```python
from build123d import *

# Parameters (mm, degrees)
SKETCH1_W           = 20
SKETCH1_H           = 20
BOSS_EXTRUDE1_DEPTH = 3
SKETCH2_W           = 14.5
SKETCH2_H           = 14.5
CUT_EXTRUDE1_DEPTH  = 3
SKETCH3_W           = 1.5
SKETCH3_H           = 3
BOSS_EXTRUDE2_DEPTH = 3
CHAMFER1_SIZE       = 1
SKETCH4_W           = 20
SKETCH4_H           = 20
SKETCH4_W_2         = 16
SKETCH4_H_2         = 16
BOSS_EXTRUDE3_DEPTH = 7
CHAMFER2_SIZE       = 1


with BuildPart() as part:
    # Sketch1 → Boss-Extrude1 (new body)
    with BuildSketch(Plane(origin=(0, 0, 0), x_dir=(1, 0, 0), z_dir=(0, 1, 0))):
        Rectangle(SKETCH1_W, SKETCH1_H)
    extrude(amount=BOSS_EXTRUDE1_DEPTH)

    # Sketch2 → Cut-Extrude1 (cut)
    with BuildSketch(Plane(origin=(0, 3, 0), x_dir=(1, 0, 0), z_dir=(0, 1, 0))):
        Rectangle(SKETCH2_W, SKETCH2_H)
    extrude(amount=-CUT_EXTRUDE1_DEPTH, mode=Mode.SUBTRACT)

    # Sketch3 → Boss-Extrude2 (add)
    with BuildSketch(Plane(origin=(0, 3, 0), x_dir=(1, 0, 0), z_dir=(0, 1, 0))):
        with Locations((6.5, 0)):
            Rectangle(SKETCH3_W, SKETCH3_H)
        with Locations((-6.5, 0)):
            Rectangle(SKETCH3_W, SKETCH3_H)
    extrude(amount=-BOSS_EXTRUDE2_DEPTH)

    # Chamfer1
    chamfer1_edges = [part.edges().sort_by_distance(p)[0] for p in [
        (5.75, 3, 0),
        (-5.75, 3, 0),
    ]]
    chamfer(chamfer1_edges, length=CHAMFER1_SIZE)

    # Sketch4 → Boss-Extrude3 (add)
    with BuildSketch(Plane.XZ):
        Rectangle(SKETCH4_W, SKETCH4_H)
        Rectangle(SKETCH4_W_2, SKETCH4_H_2, mode=Mode.SUBTRACT)
    extrude(amount=BOSS_EXTRUDE3_DEPTH)

    # Chamfer2
    chamfer2_edges = [part.edges().sort_by_distance(p)[0] for p in [
        (10, -2, 10),
        (-10, -2, 10),
        (-10, -2, -10),
        (10, -2, -10),
    ]]
    chamfer(chamfer2_edges, length=CHAMFER2_SIZE)


solid = part.part
```
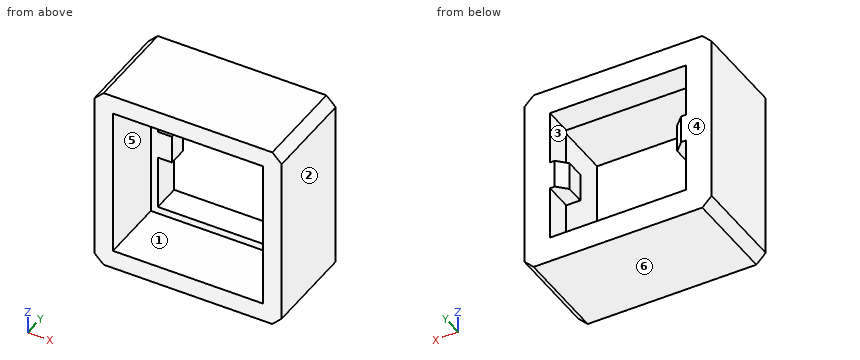
Model file for the job. Use its own axes, mm. Face numbers are marked on the shaded views. A direction names the side the tool comes from. Coordinates: 2 decimals unless noted, no trailing zeros. Write each loop counter-clockwise with the first axis right and the second up, starting at its lowest first coordinate (ties: lowest second). Pieces come first, ordered by that corner, then holes. Notation, with made-up numbers: (75, 26.25) - (118, 26.25) arc R29 cw to (118, 47.25) - close; hole circle Ø9 at (13.25, 53.5). An arc over 180 degrees is marked (long way). One line per item, written item: value. Start each with the question number.
1. Probe line 1 (Z direction, x = 5.75, y = -2); line 2 (X direction, y = 0.5, z = -2.5). List the from-to ranges inside material, lowest first. Write a range as from..to.
2. Flat gauge pin, fed straight in: pin 1 (5 mm diameter, centred on x = 3.5, z = 0, fed in from -Y). Where does the tip first touch, or does it go through?
3. Tool access for the marked faces 1, 2 and 3: list every direction of +Z, -Z, +X, -X, +Y, -Y with a clear straight run to the whole face (end or side of a thin tool).
4. Slice it at A-A (x = 0.25). Write the cut outline in (y, z).
5. Mould opens along Z. For the marked faces 4, 5 and 6 say: released by +Z, released by -Z, zero draft, split by the parting line, or undercut.
6. Slice it at B-B (y = 1.5). Write the cut outline in (x, z), plus the area to 3 significant figures.
7. Slice it at D-D (z = 3.25). Write the cut outline in (x, y).
8. Slice it at C-C (z = -0.25). Write the cut outline in (x, y), plus the area to 3 significant figures.
Answers below:
1. line 1: z = -10..-8, 8..10
1. line 2: x = -10..-7.25, 7.25..10
2. pin 1: stops at y = 0
3. face 1: -Y
3. face 2: +Z, -Z, +X, +Y, -Y
3. face 3: +Y, -Y
4. outline: (-7, -10) - (3, -10) - (3, -7.25) - (0, -7.25) - (0, -8) - (-7, -8) - close; (-7, 8) - (0, 8) - (0, 7.25) - (3, 7.25) - (3, 10) - (-7, 10) - close
5. face 4: zero draft
5. face 5: undercut
5. face 6: released by -Z
6. outline: (-10, -9) - (-9, -10) - (9, -10) - (10, -9) - (10, 9) - (9, 10) - (-9, 10) - (-10, 9) - close; hole (-7.25, -7.25) - (7.25, -7.25) - (7.25, -1.5) - (5.75, -1.5) - (5.75, 1.5) - (7.25, 1.5) - (7.25, 7.25) - (-7.25, 7.25) - (-7.25, 1.5) - (-5.75, 1.5) - (-5.75, -1.5) - (-7.25, -1.5) - close
6. area: 197 mm^2
7. outline: (-10, -7) - (-8, -7) - (-8, 0) - (-7.25, 0) - (-7.25, 3) - (-10, 3) - close; (7.25, 0) - (8, 0) - (8, -7) - (10, -7) - (10, 3) - (7.25, 3) - close
8. outline: (-10, -7) - (-8, -7) - (-8, 0) - (-5.75, 0) - (-5.75, 2) - (-6.75, 3) - (-10, 3) - close; (5.75, 0) - (8, 0) - (8, -7) - (10, -7) - (10, 3) - (6.75, 3) - (5.75, 2) - close
8. area: 52.5 mm^2
